Design review of the part built by this model. Coordinates are the model's own, in mm. Face numbers are marked on the shaded views. A direction names the side the tool comes from. Coordinates: 2 decimals unless noted, no trailing zeros. Loops run counter-clockwise (first coordinate to the right, second up) from the corner with the lowest first, then second, coordinate; pieces in that order, holes last. Notation, with made-up numbers: M -3.5,67.25 L 53.5,67.25 A12 ccw 53.5,73.25 Z; hole C 17.25,-12 d7. An arc over 180 degrees is marked long. One line per item, written item: value.
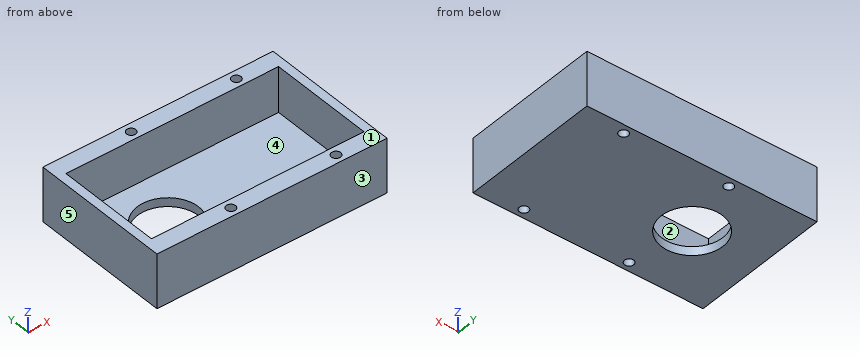
```python
from build123d import *

# Parameters (mm, degrees)
SKETCH_1_W          = 52.5
SKETCH_1_H          = 32
EXTRUDE_1_DEPTH     = 2
SKETCH_2_W          = 52.5
SKETCH_2_H          = 32
SKETCH_2_W_2        = 48.5
SKETCH_2_H_2        = 24
EXTRUDE_2_DEPTH     = 10.34
CUT_EXTRUDE_1_REACH = 64.347
SKETCH_3_R          = 7
CUT_EXTRUDE_2_REACH = 64.71
SKETCH_4_R          = 1.05


with BuildPart() as part:
    # 草图1 → 凸台-拉伸1 (new body)
    with BuildSketch(Plane.XY):
        with Locations((26.25, 16)):
            Rectangle(SKETCH_1_W, SKETCH_1_H)
    extrude(amount=EXTRUDE_1_DEPTH)

    # 草图2 → 凸台-拉伸2 (add)
    with BuildSketch(Plane.XY.offset(2)):
        with Locations((26.25, 16)):
            Rectangle(SKETCH_2_W, SKETCH_2_H)
        with Locations((26.25, 16)):
            Rectangle(SKETCH_2_W_2, SKETCH_2_H_2, mode=Mode.SUBTRACT)
    extrude(amount=EXTRUDE_2_DEPTH)

    # 草图3 → 切除-拉伸1 (cut, up to next)
    with BuildSketch(Plane.XY.offset(2), mode=Mode.PRIVATE) as cut_extrude_1_sk1:
        with Locations((15.5, 16)):
            Circle(SKETCH_3_R)
    cut_extrude_1_tool1 = extrude(cut_extrude_1_sk1.sketch, amount=-CUT_EXTRUDE_1_REACH, mode=Mode.PRIVATE) & part.part
    add(cut_extrude_1_tool1.solids().sort_by_distance((15.5, 16, 2))[0], mode=Mode.SUBTRACT)

    # 草图4 → 切除-拉伸2 (cut, up to next)
    with BuildSketch(Plane.XY.offset(12.34), mode=Mode.PRIVATE) as cut_extrude_2_sk1:
        with Locations((18.5, 30)):
            Circle(SKETCH_4_R)
    cut_extrude_2_tool1 = extrude(cut_extrude_2_sk1.sketch, amount=-CUT_EXTRUDE_2_REACH, mode=Mode.PRIVATE) & part.part
    # 草图4 → 切除-拉伸2 (cut, up to next)
    with BuildSketch(Plane.XY.offset(12.34), mode=Mode.PRIVATE) as cut_extrude_2_sk2:
        with Locations(Location((42.5, 30, 0), (0, 0, 180))):
            Circle(SKETCH_4_R)
    cut_extrude_2_tool2 = extrude(cut_extrude_2_sk2.sketch, amount=-CUT_EXTRUDE_2_REACH, mode=Mode.PRIVATE) & part.part
    # 草图4 → 切除-拉伸2 (cut, up to next)
    with BuildSketch(Plane.XY.offset(12.34), mode=Mode.PRIVATE) as cut_extrude_2_sk3:
        with Locations((42.5, 2)):
            Circle(SKETCH_4_R)
    cut_extrude_2_tool3 = extrude(cut_extrude_2_sk3.sketch, amount=-CUT_EXTRUDE_2_REACH, mode=Mode.PRIVATE) & part.part
    # 草图4 → 切除-拉伸2 (cut, up to next)
    with BuildSketch(Plane.XY.offset(12.34), mode=Mode.PRIVATE) as cut_extrude_2_sk4:
        with Locations(Location((18.5, 2, 0), (0, 0, 180))):
            Circle(SKETCH_4_R)
    cut_extrude_2_tool4 = extrude(cut_extrude_2_sk4.sketch, amount=-CUT_EXTRUDE_2_REACH, mode=Mode.PRIVATE) & part.part
    add(cut_extrude_2_tool1.solids().sort_by_distance((18.5, 30, 12.34))[0], mode=Mode.SUBTRACT)
    add(cut_extrude_2_tool2.solids().sort_by_distance((42.5, 30, 12.34))[0], mode=Mode.SUBTRACT)
    add(cut_extrude_2_tool3.solids().sort_by_distance((42.5, 2, 12.34))[0], mode=Mode.SUBTRACT)
    add(cut_extrude_2_tool4.solids().sort_by_distance((18.5, 2, 12.34))[0], mode=Mode.SUBTRACT)


solid = part.part
```
(1) We need section D-D on y = 10. State the section outline as (x, z) points.
Reply:
outline: M 0,0 L 11.89,0 L 11.89,2 L 2,2 L 2,12.34 L 0,12.34 Z; M 19.11,0 L 52.5,0 L 52.5,12.34 L 50.5,12.34 L 50.5,2 L 19.11,2 Z
(2) Insertion check: pin 1 (1.5 mm diameter, centred on x = 19.5, y = 10.5, fed in from +Z). The pin has a flat end and moves straight along its axis. Give the tip position at first contact, or say it passes through.
Reply:
pin 1: stops at z = 2
(3) We need section C-C on z = 9.75. State the section outline as (x, y) points.
Reply:
outline: M 0,0 L 52.5,0 L 52.5,32 L 0,32 Z; hole M 2,4 L 50.5,4 L 50.5,28 L 2,28 Z; hole C 18.5,2 d2.1; hole C 18.5,30 d2.1; hole C 42.5,2 d2.1; hole C 42.5,30 d2.1
(4) Mouldability with a two-part tool opening along X and no side actions: class the marked faces 3, 4 and 5 as released by +X, released by -X, zero draft, split by the parting line, or undercut.
Reply:
face 3: zero draft
face 4: undercut
face 5: released by -X
(5) Tool access review of the marked faces 1 and 2: name each direction out of +Z, -Z, +X, -X, +Y, -Y from which nothing blocks a thin tool from reaching the whole face with its end or side.
Reply:
face 1: +Z, +X, -X, +Y, -Y
face 2: +Z
(6) We need section A-A on y = 2. State the section outline as (x, z) points.
Reply:
outline: M 0,0 L 17.45,0 L 17.45,12.34 L 0,12.34 Z; M 19.55,0 L 41.45,0 L 41.45,12.34 L 19.55,12.34 Z; M 43.55,0 L 52.5,0 L 52.5,12.34 L 43.55,12.34 Z
(7) We need section B-B on x = 15.5. State the section outline as (y, z) points.
Reply:
outline: M 0,0 L 9,0 L 9,2 L 4,2 L 4,12.34 L 0,12.34 Z; M 23,0 L 32,0 L 32,12.34 L 28,12.34 L 28,2 L 23,2 Z
(8) To check wall thickness, follow line 1 along Y through (x, z) = (18.5, 8.5); line 2 along X through (y, z) = (16.5, 4.25); line 3 along Y through (x, z) = (20, 6.25). State the ranges of each line that lie inside material, in increasing order. Write a range as [from, to].
Reply:
line 1: y = [0, 0.95], [3.05, 4], [28, 28.95], [31.05, 32]
line 2: x = [0, 2], [50.5, 52.5]
line 3: y = [0, 4], [28, 32]
